Design review of the part shown in the three views and the two pictorial views. Dimensions are in mm from the part's minimum x, y and z. A direction names the side the tool comes from. Give positions to 0.01 mm unless a question says otherwise; leave off trailing zeros. Order: outer loops, then holes, each group sorted by start corner. A loop starts at its lowest first (then second) coordinate and runs counter-clockwise, first axis right, second up.
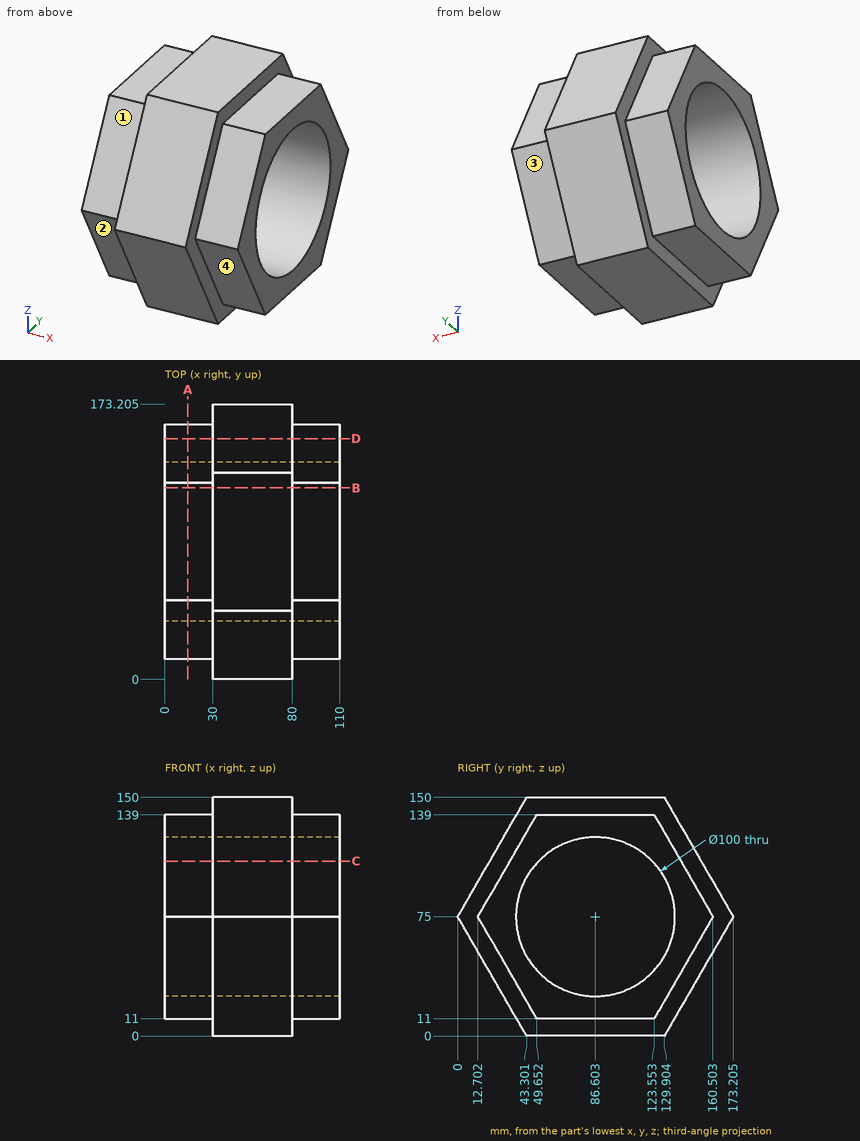
1) We need section C-C on z = 110. Give the boundary of the cut face in (x, y) (1 decimal).
Answer sheet:
outline: (0, 32.9) - (30, 32.9) - (30, 20.2) - (80, 20.2) - (80, 32.9) - (110, 32.9) - (110, 50.9) - (0, 50.9) - close; (0, 122.3) - (110, 122.3) - (110, 140.3) - (80, 140.3) - (80, 153) - (30, 153) - (30, 140.3) - (0, 140.3) - close
2) We need section B-B on y = 120.5. Give the boundary of the cut face in (x, z) (1 decimal).
Answer sheet:
outline: (0, 11) - (30, 11) - (30, 0) - (80, 0) - (80, 11) - (110, 11) - (110, 38.2) - (0, 38.2) - close; (0, 111.8) - (110, 111.8) - (110, 139) - (80, 139) - (80, 150) - (30, 150) - (30, 139) - (0, 139) - close
3) Clearance check with flat-ended pins moving along their axes: pin 1 (3 mm diameter, centred on x = 30, z = 71, fed in from +Y); pin 2 (6 mm diameter, centred on x = 17, z = 90.5, fed in from +Y); pin 3 (24 mm diameter, centred on x = 15, y = 92, fed in from -Z). State where each tip first meets the part, or that it passes through.
Answer sheet:
pin 1: stops at y = 171.76
pin 2: stops at y = 153.29
pin 3: stops at z = 11
4) We need section D-D on y = 151.5. Give the boundary of the cut face in (x, z) (1 decimal).
Answer sheet:
outline: (0, 59.4) - (30, 59.4) - (30, 37.4) - (80, 37.4) - (80, 59.4) - (110, 59.4) - (110, 90.6) - (80, 90.6) - (80, 112.6) - (30, 112.6) - (30, 90.6) - (0, 90.6) - close
5) To check wall thickness, follow line 1 (X direction, y = 155.5, z = 63); line 2 (Y direction, x = 61, z = 80.5) (1 decimal); line 3 (Y direction, x = 9, z = 54) (1 decimal). State the ranges of each line that lie inside material, in increasing order.
Answer sheet:
line 1: x = 30 to 80
line 2: y = 3.2 to 36.9, 136.3 to 170
line 3: y = 24.8 to 41.2, 132 to 148.4
6) Tool access review of the marked faces 1, 2, 3 and 4: name each direction out of +Z, -Z, +X, -X, +Y, -Y from which nothing blocks a thin tool from reaching the whole face with its end or side.
Answer sheet:
face 1: +Z, -X, -Y
face 2: -Z, -X, -Y
face 3: -Z, +X, +Y
face 4: -Z, +X, -Y
7) We need section A-A on x = 14.5. Give the boundary of the cut face in (y, z).
Answer sheet:
outline: (12.7, 75) - (49.65, 11) - (123.55, 11) - (160.5, 75) - (123.55, 139) - (49.65, 139) - close; hole circle Ø100 at (86.6, 75)
